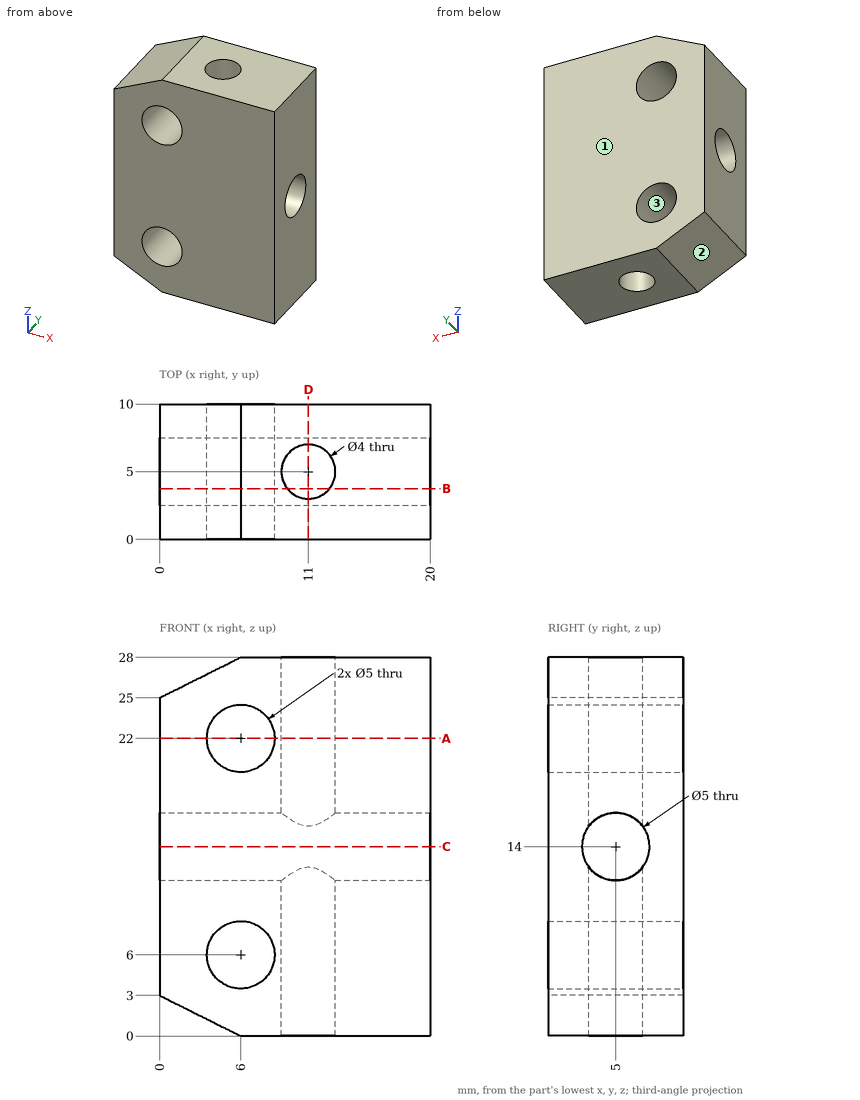
Geometry: see drawing. Coordinates: mm, zero at the bounding-box minimum. Round coordinates to 2 decimals unless told otherwise and drop trailing zeros. Write each loop counter-clockwise with the first axis right and the second up, starting at its lowest first coordinate (ties: lowest second). Pieces come first, ordered by that corner, then holes. Notation, with made-up numbers: M -22.75,10 L -9.75,10 A22 cw -9.75,37 Z; hole C 33,73.25 d3. An arc over 180 degrees is marked long. Answer in a Markdown table with one row per item. Add a question column.
(1) Cut plane A-A, the plane z = 22. Return the cut outline in (x, y).
(2) Draft query along Z for the marked faces 1, 2 and 3. Return one class per face: pulls with the +Z half, pulls with the -Z half, needs draft (parallel to the pull), parting line crosses it, or undercut.
(3) Cut plane B-B, the plane y = 3.75. Return the cut outline in (x, z).
(4) Cut plane C-C, the plane z = 14. Return the cut outline in (x, y), then the cut area to 3 significant figures.
(5) Ray query, L1, parallel to Y at x = 11, z = 4; L2, parallel to Z at x = 7, y = 6; L3, parallel to Z at x = 16.5, y = 5.5. Return the intervals inside material, ascending.
(6) Cut plane D-D, the plane x = 11. Return the cut outline in (y, z), then the cut area to 3 significant figures.
Established:
| question | item | result |
|---|---|---|
| 1 | outline | M 0,0 L 3.5,0 L 3.5,10 L 0,10 Z; M 8.5,0 L 20,0 L 20,10 L 8.5,10 Z; hole C 11,5 d4 |
| 2 | face 1 | needs draft |
| 2 | face 2 | pulls with the -Z half |
| 2 | face 3 | undercut |
| 3 | outline | M 0,3 L 6,0 L 9.44,0 L 9.44,11.83 L 0,11.83 Z; M 0,16.17 L 9.44,16.17 L 9.44,28 L 6,28 L 0,25 Z; M 12.56,0 L 20,0 L 20,11.83 L 12.56,11.83 Z; M 12.56,16.17 L 20,16.17 L 20,28 L 12.56,28 Z; hole C 6,6 d5; hole C 6,22 d5 |
| 4 | outline | M 0,0 L 20,0 L 20,2.5 L 0,2.5 Z; M 0,7.5 L 20,7.5 L 20,10 L 0,10 Z |
| 4 | area | 100 mm² |
| 5 | L1 | 0 to 3, 7 to 10 |
| 5 | L2 | 0 to 3.71, 8.29 to 11.71, 16.29 to 19.71, 24.29 to 28 |
| 5 | L3 | 0 to 11.55, 16.45 to 28 |
| 6 | outline | M 0,0 L 3,0 L 3,12.5 A2.5 cw 3,15.5 L 3,28 L 0,28 Z; M 7,0 L 10,0 L 10,28 L 7,28 L 7,15.5 A2.5 cw 7,12.5 Z |
| 6 | area | 166 mm² |
